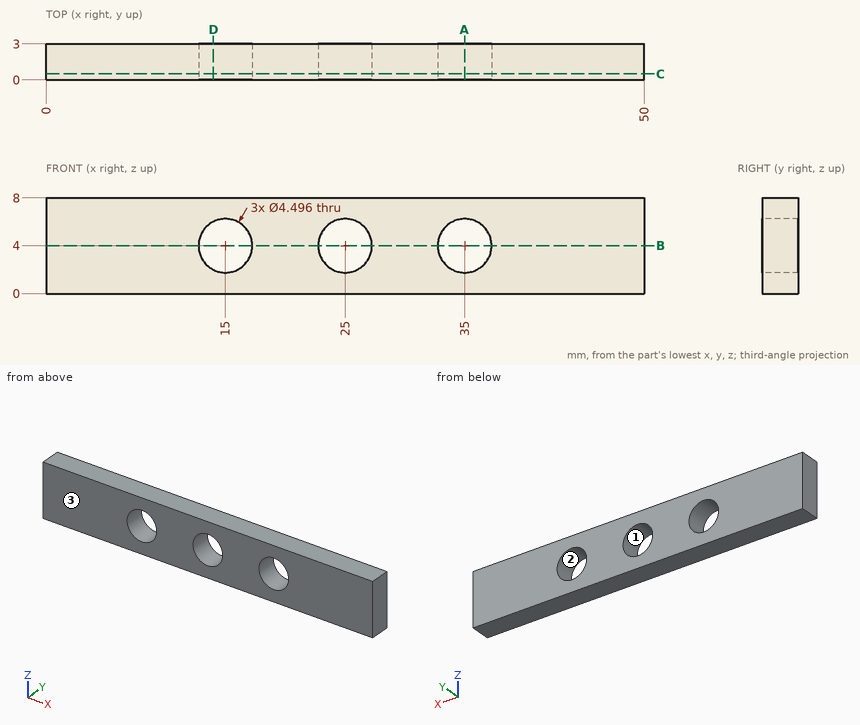
Geometry check sheet. Reference: drawing and pictorial views, mm from the part's lowest x, y, z. Round coordinates to 2 decimals unless told otherwise and drop trailing zeros. Loops run counter-clockwise (first coordinate to the right, second up) from the corner with the lowest first, then second, coordinate; pieces in that order, holes last.
1. Sectioned sample at A-A on x = 35. Record the boundary of the cut face in (y, z).
2. Sectioned sample at D-D on x = 14. Record the boundary of the cut face in (y, z).
3. Sectioned sample at C-C on y = 0.5. Record the boundary of the cut face in (x, z), and give its area (3 significant figures).
4. Sectioned sample at B-B on z = 4. Record the boundary of the cut face in (x, y).
5. Gauge pin test, flat end, axial feed: pin 1 Ø4 at (x, z) = (25, 4) entering from -Y. Record the tip position at first contact, or that the pin passes through.
6. Scan lines: probe 1 along X at (y, z) = (2.85, 4); probe 2 along Z at (x, y) = (17, 2.3) (1 decimal); probe 3 along X at (y, z) = (0.6, 5.5) (1 decimal). Record each from-to range of solid material in increasing order.
7. Mould release check, pull along X, two halves, no side actions. Record for the marked faces 1, 2 and 3: released by +X, released by -X, zero draft, split by the parting line, or undercut.
Recorded:
1. outline: (0, 0) - (3, 0) - (3, 1.75) - (0, 1.75) - close; (0, 6.25) - (3, 6.25) - (3, 8) - (0, 8) - close
2. outline: (0, 0) - (3, 0) - (3, 1.99) - (0, 1.99) - close; (0, 6.01) - (3, 6.01) - (3, 8) - (0, 8) - close
3. outline: (0, 0) - (50, 0) - (50, 8) - (0, 8) - close; hole circle Ø4.5 at (15, 4); hole circle Ø4.5 at (25, 4); hole circle Ø4.5 at (35, 4)
3. area: 352 mm2
4. outline: (0, 0) - (12.75, 0) - (12.75, 3) - (0, 3) - close; (17.25, 0) - (22.75, 0) - (22.75, 3) - (17.25, 3) - close; (27.25, 0) - (32.75, 0) - (32.75, 3) - (27.25, 3) - close; (37.25, 0) - (50, 0) - (50, 3) - (37.25, 3) - close
5. pin 1: passes through
6. probe 1: x = 0 to 12.75, 17.25 to 22.75, 27.25 to 32.75, 37.25 to 50
6. probe 2: z = 0 to 3, 5 to 8
6. probe 3: x = 0 to 13.3, 16.7 to 23.3, 26.7 to 33.3, 36.7 to 50
7. face 1: undercut
7. face 2: undercut
7. face 3: zero draft
